from build123d import *

# Parameters (mm, degrees)
F1_DEPTH  = 12.7
F2_W      = 12.7
F2_H      = 12.7
F3_DEPTH  = 12.7
F5_W      = 10.16
F5_H      = 5.08
F6_DEPTH  = 12.7
F7_W      = 5.08
F7_H      = 10.16
F8_DEPTH  = 12.7
F9_W      = 10.16
F9_H      = 10.16
F10_DEPTH = 12.7


with BuildPart() as f1:
    # F0 (on Top) → F1 (new body)
    with BuildSketch(Plane.XY):
        Polygon((0, 12.7), (0, 0), (25.4, 0), (25.4, 12.7), (25.4, 25.4), (12.7, 25.4), (12.7, 12.7), align=None)
    extrude(amount=F1_DEPTH)

    # F2 (on face) → F3 (join)
    with BuildSketch(Plane.XY.offset(12.7)):
        with Locations((19.05, 6.35)):
            Rectangle(F2_W, F2_H)
    extrude(amount=F3_DEPTH)

    # F5 (on face) → F6 (cut)
    with BuildSketch(Plane.XY.offset(25.4)):
        with Locations((19.05, 3.81)):
            Rectangle(F5_W, F5_H)
        with BuildLine():
            Line((13.97, 6.35), (24.13, 6.35))
            ThreePointArc((24.13, 6.35), (19.05, 11.43), (13.97, 6.35))
        make_face()
    extrude(amount=-F6_DEPTH, mode=Mode.SUBTRACT)

    # F7 (on face) → F8 (cut)
    with BuildSketch(Plane(origin=(0, 0, 0), x_dir=(0, -1, 0), z_dir=(-1, 0, 0))):
        with Locations((-3.81, 6.35)):
            Rectangle(F7_W, F7_H)
        with BuildLine():
            Line((-6.35, 1.27), (-6.35, 11.43))
            ThreePointArc((-6.35, 11.43), (-11.43, 6.35), (-6.35, 1.27))
        make_face()
    extrude(amount=-F8_DEPTH, mode=Mode.SUBTRACT)

    # F9 (on face) → F10 (cut)
    with BuildSketch(Plane(origin=(0, 25.4, 0), x_dir=(-1, 0, 0), z_dir=(0, 1, 0))):
        with Locations((-19.05, 6.35)):
            Rectangle(F9_W, F9_H)
    extrude(amount=-F10_DEPTH, mode=Mode.SUBTRACT)


solid = f1.part
The listing builds one solid part. Answer for the finished solid, in the listing's coordinates (mm). A direction names the side the tool comes from. Coordinates: 2 decimals unless noted, no trailing zeros. Write each loop counter-clockwise with the first axis right and the second up, starting at its lowest first coordinate (ties: lowest second). Pieces come first, ordered by that corner, then holes. Notation, with made-up numbers: (1, 8.25) -> (56, 8.25) arc R4 cw to (56, 14.25) -> close; hole circle Ø11 at (43.5, 84). An arc over 180 degrees is marked (long way). One line per question, with ' | ' between items.
1. Given pin 1 Ø5 at (x, y) = (18.5, 20) entering from -Z; pin 2 Ø1.5 at (y, z) = (12, 17.5) entering from -X; pin 3 Ø6.5 at (x, y) = (18, 18) entering from +Z; pin 4 Ø8 at (x, z) = (21, 18.5) entering from +Y, each flat-ended and moving along its own axis, determine where each tip first touches the part or whether it passes through.
Verdict:
pin 1: stops at z = 0 | pin 2: stops at x = 12.7 | pin 3: stops at z = 12.7 | pin 4: stops at y = 12.7
2. Section C-C (z = 6.35) is taken. Determine the outline of the cut face in (x, y).
Verdict:
outline: (0, 0) -> (25.4, 0) -> (25.4, 25.4) -> (24.13, 25.4) -> (24.13, 12.7) -> (13.97, 12.7) -> (13.97, 25.4) -> (12.7, 25.4) -> (12.7, 12.7) -> (0, 12.7) -> (0, 11.43) -> (12.7, 11.43) -> (12.7, 1.27) -> (0, 1.27) -> close
3. Section B-B (x = 5.5) is taken. Determine the outline of the cut face in (y, z).
Verdict:
outline: (0, 0) -> (12.7, 0) -> (12.7, 12.7) -> (0, 12.7) -> close; hole (1.27, 1.27) -> (6.35, 1.27) arc R5.08 ccw to (6.35, 11.43) -> (1.27, 11.43) -> close
4. Section A-A (z = 15.5) is taken. Determine the outline of the cut face in (x, y), and give its area (3 significant figures).
Verdict:
outline: (12.7, 0) -> (25.4, 0) -> (25.4, 12.7) -> (12.7, 12.7) -> close; hole (13.97, 1.27) -> (24.13, 1.27) -> (24.13, 6.35) arc R5.08 ccw to (13.97, 6.35) -> close | area: 69.1 mm^2
5. Straight lines are drawn through the part: line 1 (X direction, y = 16.5, z = 4.5); line 2 (Z direction, x = 18.5, y = 21.25); line 3 (X direction, y = 11, z = 7.5). For each, find the intervals that lie inside material, in ascending order.
Verdict:
line 1: x = 12.7 to 13.97, 24.13 to 25.4 | line 2: z = 0 to 1.27, 11.43 to 12.7 | line 3: x = 12.7 to 25.4
6. For a pull along Y with two mould halves and no side action, classify faces 5 (the flat face through (6, 1.27, 6)), 6 (the flat face through (19, 12.7, 19)), 7 (the flat face through (16, 11, 25.4)) as released by +Y, released by -Y, zero draft, split by the parting line, or undercut.
Verdict:
face 5: undercut | face 6: released by +Y | face 7: zero draft
7. Which of the six approach directions +Z, -Z, +X, -X, +Y, -Y give full straight-line access (tool end or side, diameter ignored) to faces 1 (the flat face through (13.97, 4, 19)), 2 (the flat face through (6, 12.7, 6)), 3 (the flat face through (19, 19, 11.43)), 4 (the flat face through (12.7, 6, 6))?
Verdict:
face 1: +Z | face 2: +Z, -Z, -X, +Y | face 3: +Y | face 4: -X
